```python
from build123d import *

# Parameters (mm, degrees)
F1_DEPTH = 12


with BuildPart() as f1:
    # F0 (on Front) → F1 (new body)
    with BuildSketch(Plane.XZ):
        with BuildLine():
            Line((-5.99854, 136.132353), (-5.99854, 189.905286))
            ThreePointArc((-5.99854, 189.905286), (-134.349772, 134.350805), (-189.90524, 6))
            Line((-189.90524, 6), (-136, 6))
            ThreePointArc((-136, 6), (-130, 0), (-136, -6))
            Line((-136, -6), (-189.90524, -6))
            ThreePointArc((-189.90524, -6), (-134.349772, -134.350805), (-5.99854, -189.905286))
            Line((-5.99854, -189.905286), (-5.99854, -136.132353))
            ThreePointArc((-5.99854, -136.132353), (-6, -136), (-5.99854, -135.867647))
            ThreePointArc((-5.99854, -135.867647), (0, -130), (5.99854, -135.867647))
            ThreePointArc((5.99854, -135.867647), (6, -136), (5.99854, -136.132353))
            Line((5.99854, -136.132353), (5.99854, -189.905286))
            ThreePointArc((5.99854, -189.905286), (134.350288, -134.350288), (189.905286, -5.99854))
            Line((189.905286, -5.99854), (136.132353, -5.99854))
            ThreePointArc((136.132353, -5.99854), (136, -6), (135.867647, -5.99854))
            ThreePointArc((135.867647, -5.99854), (130, 0), (135.867647, 5.99854))
            Line((135.867647, 5.99854), (189.905286, 5.99854))
            ThreePointArc((189.905286, 5.99854), (134.350288, 134.350288), (5.99854, 189.905286))
            Line((5.99854, 189.905286), (5.99854, 136.132353))
            ThreePointArc((5.99854, 136.132353), (6, 136), (5.99854, 135.867647))
            ThreePointArc((5.99854, 135.867647), (0, 130), (-5.99854, 135.867647))
            ThreePointArc((-5.99854, 135.867647), (-6, 136), (-5.99854, 136.132353))
        make_face()
    extrude(amount=F1_DEPTH)


solid = f1.part
```
Model file for the job. Use its own axes, mm. A direction names the side the tool comes from. Give positions to 0.01 mm unless a question says otherwise; leave off trailing zeros. Loops run counter-clockwise (first coordinate to the right, second up) from the corner with the lowest first, then second, coordinate; pieces in that order, holes last. Notation, with made-up numbers: (47, -13.5) - (79, -13.5) arc R21 cw to (79, 12.5) - close; hole circle Ø6 at (41.25, 10.5). An arc over 180 degrees is marked (long way). One line per item, written item: value. Start each with the question number.
1. Slice it at C-C (z = 0). List the corners of the cut face in (x, y), plus the area to 3 significant figures.
2. Slice it at B-B (x = 0). List the corners of the cut face in (y, z).
3. Pin check, flat tips, straight feed: pin 1 (1 mm diameter, centred on y = -8.5, z = -33, fed in from +X); pin 2 (4 mm diameter, centred on y = -1.5, z = -140.5, fed in from -X); pin 3 (6 mm diameter, centred on y = -7, z = -176, fed in from +X). Stop position of each tip, or through.
4. Slice it at A-A (y = -7). List the corners of the cut face in (x, z), plus the area to 3 significant figures.
5. Which spindle directions (+Z, -Z, +X, -X, +Y, -Y) get a long thin tool onto all of the face, cutting with end or side? Do faces 4 (the flat face through (-5.999, -6, 163)), 5 (the flat face through (5.999, -6, -163)), 6 (the flat face through (163, -6, -5.999)), 7 (the flat face through (-163, -6, -6)), 8 (the flat face through (-3, -12, 3)). Say none if no direction does.
6. Pull direction Z, two halves, no side cores. Call faces 1 (the flat face through (-163, -6, 6)), 2 (the cylindrical face through (132.925, -5.916, -135.761)), 3 (the flat face through (5.999, -6, 163)): pulls with the +Z half, pulls with the -Z half, needs draft (parallel to the pull), parting line crosses it, or undercut.
7. Probe L1, parallel to X at y = -9, z = 144.5; L2, parallel to X at y = -5.75, z = 151.5; L3, parallel to X at y = -0.25, z = 72.5. List the from-to ranges inside material, lowest first. Write a range as from..to.
Solution:
1. outline: (-130, -12) - (130, -12) - (130, 0) - (-130, 0) - close
1. area: 3,120 mm^2
2. outline: (-12, -130) - (0, -130) - (0, 130) - (-12, 130) - close
3. pin 1: stops at x = 187.2
3. pin 2: stops at x = -130.07
3. pin 3: stops at x = 78.56
4. outline: (-189.91, -6) arc R190 ccw to (-6, -189.91) - (-6, -136.13) arc R6 cw to (-6, -135.87) arc R6 cw to (6, -135.87) arc R6 cw to (6, -136.13) - (6, -189.91) arc R190 ccw to (189.91, -6) - (136.13, -6) arc R6 cw to (135.87, -6) arc R6 cw to (135.87, 6) - (189.91, 6) arc R190 ccw to (6, 189.91) - (6, 136.13) arc R6 cw to (6, 135.87) arc R6 cw to (-6, 135.87) arc R6 cw to (-6, 136.13) - (-6, 189.91) arc R190 ccw to (-189.91, 6) - (-136, 6) arc R6 cw to (-136, -6) - close
4. area: 111,000 mm^2
5. face 4: +Z, +Y, -Y
5. face 5: -Z, +Y, -Y
5. face 6: +X, +Y, -Y
5. face 7: -X, +Y, -Y
5. face 8: +Z, -Z, +X, -X, -Y
6. face 1: undercut
6. face 2: pulls with the -Z half
6. face 3: needs draft
7. L1: x = -123.37..-6, 6..123.37
7. L2: x = -114.66..-6, 6..114.66
7. L3: x = -175.62..175.62
